Could you check a few things on this model? Use its own coordinates, in mm. Face numbers are marked on the shaded views. A direction names the side the tool comes from. Coordinates: 2 decimals unless noted, no trailing zeros. Loops run counter-clockwise (first coordinate to the right, second up) from the corner with the lowest first, then second, coordinate; pieces in that order, holes last. Notation, with made-up numbers: M -26.75,75 L 18.25,75 A8 cw 18.25,85 Z; hole C 69,46 d5. An arc over 180 degrees is marked long. Return JSON: item names as keys, results as strings. Group by question number.
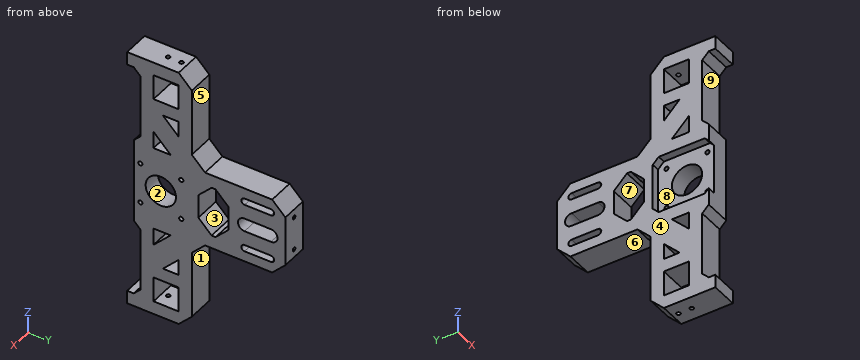
from build123d import *

# Parameters (mm, degrees)
SKETCH1_W           = 100
SKETCH1_H           = 120
BOSS_EXTRUDE1_DEPTH = 20
SKETCH2_W           = 19.05
SKETCH2_H           = 19.05
CUT_EXTRUDE1_DEPTH  = 20
SKETCH3_R           = 1.5
CUT_EXTRUDE2_DEPTH  = 20
SKETCH5_R           = 11.5
SKETCH5_R_2         = 1.6
CUT_EXTRUDE3_DEPTH  = 20
SKETCH6_W           = 44
SKETCH6_H           = 44
MOTOR_INDENT_DEPTH  = 6
BEARING_BLOCK_DEPTH = 21
SKETCH8_W           = 71
SKETCH8_H           = 70.95
CUT_EXTRUDE6_DEPTH  = 21
CHAMFER1_SIZE       = 10
SKETCH10_W          = 58
SKETCH10_H          = 10
CUT_EXTRUDE7_DEPTH  = 21
CHAMFER2_SIZE       = 5
CHAMFER3_SIZE       = 4.5
SKETCH11_R          = 1.45
CUT_EXTRUDE8_DEPTH  = 10
SKETCH12_W          = 38
SKETCH12_H          = 23
CUT_EXTRUDE9_DEPTH  = 21
CHAMFER4_SIZE       = 10
CUT_EXTRUDE10_DEPTH = 21
SKETCH14_W          = 64
SKETCH14_H          = 5
CUT_EXTRUDE11_DEPTH = 21


with BuildPart() as part:
    # Sketch1 → Boss-Extrude1 (new body)
    with BuildSketch(Plane(origin=(0, 0, 0), x_dir=(0, 0, -1), z_dir=(1, 0, 0))):
        with Locations((-50, 60)):
            Rectangle(SKETCH1_W, SKETCH1_H)
    boss_extrude1 = extrude(amount=BOSS_EXTRUDE1_DEPTH)

    # Sketch2 → Cut-Extrude1 (cut)
    with BuildSketch(Plane(origin=(20, 0, 0), x_dir=(0, 0, -1), z_dir=(1, 0, 0))):
        with Locations((-80.475, 29.525)):
            Rectangle(SKETCH2_W, SKETCH2_H)
    cut_extrude1 = extrude(amount=-CUT_EXTRUDE1_DEPTH, mode=Mode.SUBTRACT)

    # Sketch3 → Cut-Extrude2 (cut)
    with BuildSketch(Plane.XY.offset(100)):
        with Locations((10, 34.605)):
            Circle(SKETCH3_R)
        with Locations((10, 24.445)):
            Circle(SKETCH3_R)
    cut_extrude2 = extrude(amount=-CUT_EXTRUDE2_DEPTH, mode=Mode.SUBTRACT)

    # Mirror1: Boss-Extrude1, Cut-Extrude1, Cut-Extrude2 across plane
    add(boss_extrude1.mirror(Plane(origin=(20, 0, 0), x_dir=(1, 0, 0), z_dir=(0, 0, 1))))
    add(cut_extrude1.mirror(Plane(origin=(20, 0, 0), x_dir=(1, 0, 0), z_dir=(0, 0, 1))), mode=Mode.SUBTRACT)
    add(cut_extrude2.mirror(Plane(origin=(20, 0, 0), x_dir=(1, 0, 0), z_dir=(0, 0, 1))), mode=Mode.SUBTRACT)

    # Sketch5 → Cut-Extrude3 (cut)
    with BuildSketch(Plane(origin=(20, 0, 0), x_dir=(0, 0, -1), z_dir=(1, 0, 0))):
        with Locations((0, 25.5)):
            Circle(SKETCH5_R)
        with Locations((-15.5, 41)):
            Circle(SKETCH5_R_2)
        with Locations((15.5, 41)):
            Circle(SKETCH5_R_2)
        with Locations((15.5, 10)):
            Circle(SKETCH5_R_2)
        with Locations((-15.5, 10)):
            Circle(SKETCH5_R_2)
    extrude(amount=-CUT_EXTRUDE3_DEPTH, mode=Mode.SUBTRACT)

    # Sketch6 → Motor indent (cut)
    with BuildSketch(Plane.ZY):
        with Locations((0, 25.5)):
            Rectangle(SKETCH6_W, SKETCH6_H)
    extrude(amount=-MOTOR_INDENT_DEPTH, mode=Mode.SUBTRACT)

    # Sketch7 → Bearing Block (cut, through all)
    with BuildSketch(Plane.ZY):
        with BuildLine():
            Line((5, 109.05), (5, 89.05))
            ThreePointArc((5, 89.05), (0, 84.05), (-5, 89.05))
            Line((-5, 89.05), (-5, 109.05))
            ThreePointArc((-5, 109.05), (0, 114.05), (5, 109.05))
        make_face()
        with BuildLine():
            Line((-16, 109.05), (-16, 89.05))
            ThreePointArc((-16, 89.05), (-18.5, 86.55), (-21, 89.05))
            Line((-21, 89.05), (-21, 109.05))
            ThreePointArc((-21, 109.05), (-18.5, 111.55), (-16, 109.05))
        make_face()
        with BuildLine():
            Line((16, 109.05), (16, 89.05))
            ThreePointArc((16, 89.05), (18.5, 86.55), (21, 89.05))
            Line((21, 89.05), (21, 109.05))
            ThreePointArc((21, 109.05), (18.5, 111.55), (16, 109.05))
        make_face()
    extrude(amount=-BEARING_BLOCK_DEPTH, mode=Mode.SUBTRACT)

    # Sketch8 → Cut-Extrude6 (cut, through all)
    with BuildSketch(Plane(origin=(20, 0, 0), x_dir=(0, 0, -1), z_dir=(1, 0, 0))):
        with Locations((-64.5, 84.525)):
            Rectangle(SKETCH8_W, SKETCH8_H)
        with Locations((64.5, 84.525)):
            Rectangle(SKETCH8_W, SKETCH8_H)
    extrude(amount=-CUT_EXTRUDE6_DEPTH, mode=Mode.SUBTRACT)

    # Chamfer1
    chamfer1_edges = [part.edges().sort_by_distance(p)[0] for p in [
        (10, 120, 29),
        (10, 49.05, 29),
        (10, 49.05, 100),
        (10, 49.05, -100),
        (10, 49.05, -29),
        (10, 120, -29),
    ]]
    chamfer(chamfer1_edges, length=CHAMFER1_SIZE)

    # Sketch10 → Cut-Extrude7 (cut, through all)
    with BuildSketch(Plane.ZY):
        with Locations((-61, 5)):
            Rectangle(SKETCH10_W, SKETCH10_H)
        with Locations((61, 5)):
            Rectangle(SKETCH10_W, SKETCH10_H)
    extrude(amount=-CUT_EXTRUDE7_DEPTH, mode=Mode.SUBTRACT)

    # Chamfer2
    chamfer2_edges = [part.edges().sort_by_distance(p)[0] for p in [
        (10, 10, -90),
        (10, 10, -32),
        (10, 10, 32),
        (10, 10, 90),
    ]]
    chamfer(chamfer2_edges, length=CHAMFER2_SIZE)

    # Chamfer3
    chamfer3_edges = [part.edges().sort_by_distance(p)[0] for p in [
        (3, 47.5, 22),
        (3, 3.5, 22),
        (3, 3.5, -22),
        (3, 47.5, -22),
    ]]
    chamfer(chamfer3_edges, length=CHAMFER3_SIZE)

    # Sketch11 → Cut-Extrude8 (cut)
    with BuildSketch(Plane(origin=(0, 120, 0), x_dir=(1, 0, 0), z_dir=(0, 1, 0))):
        with Locations((10, -12.7)):
            Circle(SKETCH11_R)
        with Locations((10, 12.7)):
            Circle(SKETCH11_R)
    extrude(amount=-CUT_EXTRUDE8_DEPTH, mode=Mode.SUBTRACT)

    # Sketch12 → Cut-Extrude9 (cut, through all)
    with BuildSketch(Plane(origin=(20, 0, 0), x_dir=(0, 0, -1), z_dir=(1, 0, 0))):
        with Locations((0, 65.55)):
            Rectangle(SKETCH12_W, SKETCH12_H)
    extrude(amount=-CUT_EXTRUDE9_DEPTH, mode=Mode.SUBTRACT)

    # Chamfer4
    chamfer4_edges = [part.edges().sort_by_distance(p)[0] for p in [
        (10, 54.05, 19),
        (10, 77.05, 19),
        (10, 77.05, -19),
        (10, 54.05, -19),
    ]]
    chamfer(chamfer4_edges, length=CHAMFER4_SIZE)

    # Sketch13 → Cut-Extrude10 (cut, through all)
    with BuildSketch(Plane.ZY):
        Polygon((-49, 39.05), (-60.95, 27.1), (-60.95, 39.05), align=None)
        Polygon((-32, 33), (-45, 20), (-32, 20), align=None)
    cut_extrude10 = extrude(amount=-CUT_EXTRUDE10_DEPTH, mode=Mode.SUBTRACT)

    # Mirror2: Cut-Extrude10 across plane
    add(cut_extrude10.mirror(Plane.XY), mode=Mode.SUBTRACT)

    # Sketch14 → Cut-Extrude11 (cut, through all)
    with BuildSketch(Plane(origin=(20, 0, 0), x_dir=(0, 0, -1), z_dir=(1, 0, 0))):
        with Locations((0, 2.5)):
            Rectangle(SKETCH14_W, SKETCH14_H)
    extrude(amount=-CUT_EXTRUDE11_DEPTH, mode=Mode.SUBTRACT)


solid = part.part
(1) For the marked faces 5, 6, 7, 8 and 9, which set-ups out of +Z, -Z, +X, -X, +Y, -Y let a thin tool reach every point of the face, with its end or its side?
(2) We'd pull the mould along Y, two halves only. Please class the marked faces 1, 2, 3 and 4: +Y half, -Y half, draft (parallel to the pull), parting line (faces both ways), or undercut.
(3) Imagine slicing it at D-D, the plane x = 3.25. Count the separate pieces of the cut face and the enclosed holes in it, then the cut area to 3 significant figures.
(4) Imagine slicing it at B-B, the plane y = 91. Write out the boundary of the cut face in (x, z), then the cut area to 3 significant figures.
(5) Imagine slicing it at A-A, the plane z = -55. Write out the boundary of the cut face in (x, y), then the cut area to 3 significant figures.
(6) If I drill on L1, parallel to Z at x = 13.75, y = 93; L2, parallel to Z at x = 19.25, y = 41.5; L3, parallel to Y at x = 15, z = 18, over which ranges is the centre line in solid material (lowest first)? Write a range as [from, to].
(7) Will these pins go through, and if not, where does the flat tip stop? P1, Ø6.5, axis at x = 11.5, z = -40.5, coming from the +Y side; P2, Ø3, axis at y = 41, z = -15.5, coming from the -X side; P3, Ø5, axis at x = 9.5, y = 70.5, coming from the -Z side; P4, Ø1.7, axis at x = 10, z = -12.7, coming from the +Y side.
(8) Imagine slicing it at C-C, the plane z = 0. Write out the boundary of the cut face in (x, y), then the cut area to 3 significant figures.
Checks:
{
 "1": {"face 5": "+Z, +X, -X, +Y", "face 6": "-Z, +X, -X, +Y", "face 7": "+X, -X", "face 8": "-X", "face 9": "+X, -X, -Y"},
 "2": {"face 1": "+Y half", "face 2": "undercut", "face 3": "undercut", "face 4": "draft"},
 "3": {"separate pieces": "1", "enclosed holes": "10", "area": "8,320 mm²"},
 "4": {"outline": "M 0,-29 L 20,-29 L 20,-21 L 0,-21 Z; M 0,-16 L 20,-16 L 20,-5 L 0,-5 Z; M 0,5 L 20,5 L 20,16 L 0,16 Z; M 0,21 L 20,21 L 20,29 L 0,29 Z", "area": "760 mm²"},
 "5": {"outline": "M 0,10 L 20,10 L 20,33.05 L 0,33.05 Z; M 0,39.05 L 20,39.05 L 20,49.05 L 0,49.05 Z", "area": "661 mm²"},
 "6": {"L1": "[-29, -21], [-16, -5], [5, 16], [21, 29]", "L2": "[-97.55, -17.02], [-13.98, 13.98], [17.02, 97.55]", "L3": "[5, 63.05], [68.05, 86.6], [111.5, 120]"},
 "7": {"P1": "y = 50.8", "P2": "through", "P3": "z = -29", "P4": "y = 110"},
 "8": {"outline": "M 0,47.5 L 6,47.5 L 6,37 L 20,37 L 20,54.05 L 0,54.05 Z; M 0,77.05 L 20,77.05 L 20,84.05 L 0,84.05 Z; M 0,114.05 L 20,114.05 L 20,120 L 0,120 Z; M 6,5 L 20,5 L 20,14 L 6,14 Z", "area": "663 mm²"}
}
